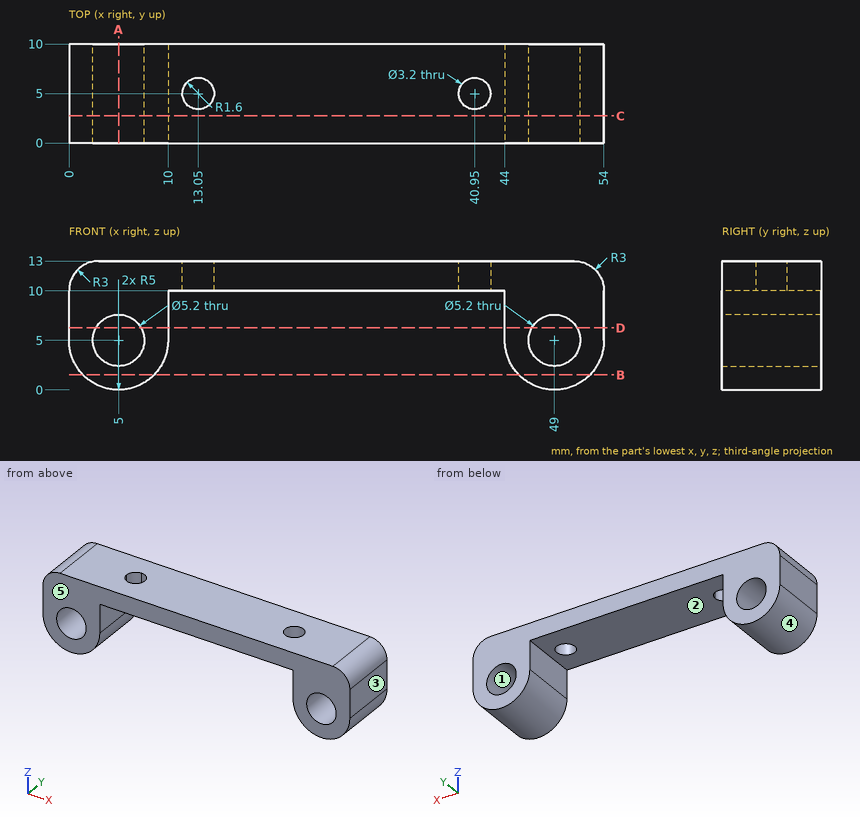
Job drawing, mm, ordinate dimensions from the low corner. One solid piece. A direction names the side the tool comes from. Round coordinates to 2 decimals unless told otherwise and drop trailing zeros. Loops run counter-clockwise (first coordinate to the right, second up) from the corner with the lowest first, then second, coordinate; pieces in that order, holes last. Notation, with made-up numbers: M 6.25,56.25 L 65.25,56.25 A18 cw 65.25,80.25 Z; hole C 41.5,-15 d10. An arc over 180 degrees is marked long. Answer as CSV lines item,"result".
1. Flat gauge pins, fed straight in: P1, Ø7, axis at x = 5, z = 5, coming from the +Y side; P2, Ø4, axis at x = 40.95, y = 5, coming from the -Z side. Where does each tip first touch, or does it go through?
Resolved:
P1,"stops at y = 10"
P2,"stops at z = 10"
2. Two-plate mould, pull along X, no slides. Class the marked faces 3, 4 and 5: released by +X, released by -X, zero draft, split by the parting line, or undercut.
Resolved:
face 3,"released by +X"
face 4,"undercut"
face 5,"zero draft"
3. Cut at B-B on z = 1.5. Write the cut outline in (x, y).
Resolved:
outline,"M 1.43,0 L 8.57,0 L 8.57,10 L 1.43,10 Z; M 45.43,0 L 52.57,0 L 52.57,10 L 45.43,10 Z"
4. 3-axis set-ups, long thin cutter, end or side, ignore diameter. For the marked faces 1 and 2: which of +Z, -Z, +X, -X, +Y, -Y reach the whole face in a straight line?
Resolved:
face 1,"+Y, -Y"
face 2,"-Z, +Y, -Y"
5. Cut at C-C on y = 2.75. Write the cut outline in (x, z).
Resolved:
outline,"M 0,5 A5 ccw 10,5 L 10,10 L 44,10 L 44,5 A5 ccw 54,5 L 54,10 A3 ccw 51,13 L 3,13 A3 ccw 0,10 Z; hole C 5,5 d5.2; hole C 49,5 d5.2"
6. Wall check: probe 1 along X at (y, z) = (2.75, 5); probe 2 along Y at (x, z) = (40.95, 11.75); probe 3 along X at (y, z) = (3.75, 4). Give the ranges that are in metal, low to high. Write a range as [from, to].
Resolved:
probe 1,"x = [0, 2.4], [7.6, 10], [44, 46.4], [51.6, 54]"
probe 2,"y = [0, 3.4], [6.6, 10]"
probe 3,"x = [0.1, 2.6], [7.4, 9.9], [44.1, 46.6], [51.4, 53.9]"
7. Cut at A-A on x = 5. Write the cut outline in (y, z), then the cut area to 3 significant figures.
Resolved:
outline,"M 0,0 L 10,0 L 10,2.4 L 0,2.4 Z; M 0,7.6 L 10,7.6 L 10,13 L 0,13 Z"
area,"78.0 mm²"
8. Cut at D-D on z = 6.25. Write the cut outline in (x, y), then the cut area to 3 significant figures.
Resolved:
outline,"M 0,0 L 2.72,0 L 2.72,10 L 0,10 Z; M 7.28,0 L 10,0 L 10,10 L 7.28,10 Z; M 44,0 L 46.72,0 L 46.72,10 L 44,10 Z; M 51.28,0 L 54,0 L 54,10 L 51.28,10 Z"
area,"109 mm²"
